Input: part model. Units: mm. Frame: model coordinates. Face numbers are marked on the shaded views. A direction names the side the tool comes from. Give positions to 0.01 mm unless a question says otherwise; leave off trailing zeros. Loops run counter-clockwise (first coordinate to the right, second up) from the corner with the lowest first, then second, coordinate; pieces in that order, holes last. Notation, with made-up numbers: (61, -23.75) -> (96, -23.75) arc R24 cw to (96, -11.75) -> close; hole circle Ø2 at (81, 3). An arc over 180 degrees is marked (long way). One line per question, with ' | ' between items.
from build123d import *

# Parameters (mm, degrees)
CIRPATTERN1_COUNT = 6


with BuildPart() as part:
    # Sketch1 → Revolve1 (revolve)
    with BuildSketch(Plane.XY, mode=Mode.PRIVATE) as revolve1_sk:
        Polygon((0, 16), (0, 20), (7.5, 20), (7.5, 18.5), (13, 18.5), (13, 16), (13.5, 16), (13.5, 15), (29.4, 15), (29.4, 13.95), (30.8, 13.95), (30.8, 14.8), (32.2, 14.8), (32.2, 12), (7, 12), (7, 15), (6.5, 15), (6.5, 16), align=None)
    revolve(revolve1_sk.sketch.rotate(Axis((-3.70841034, 0, 0), (1, 0, 0)), 180), axis=Axis((-3.70841034, 0, 0), (1, 0, 0)))

    # Sketch4 → M3 Tapped Hole1 (revolve, cut)
    with BuildSketch(Plane(origin=(0, 0, 18), x_dir=(0, 0, 1), z_dir=(0, 1, 0))):
        Polygon((0, 0), (0, 8.251075774), (1.25, 7.5), (1.25, 0), align=None)
    m3_tapped_hole1 = revolve(axis=Axis((-6.35, 0, 18), (1, 0, 0)), mode=Mode.SUBTRACT)

    # CirPattern1: M3 Tapped Hole1 ×6 about axis
    cirpattern1_axis = Axis((0, 0, 0), (1, 0, 0))
    for i in range(1, CIRPATTERN1_COUNT):
        add(m3_tapped_hole1.rotate(cirpattern1_axis, i * 360 / CIRPATTERN1_COUNT), mode=Mode.SUBTRACT)


solid = part.part
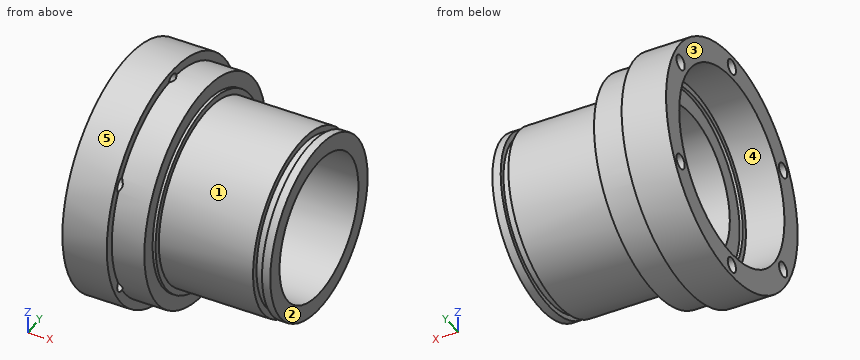
1. Section query A-A (x = 27.5). Output: boundary loops of the cut face in (y, z).
Determined:
outline: circle Ø30 at (0, 0); hole circle Ø24 at (0, 0)
2. Pull-direction query (Y, two-part tool) for the marked faces 3, 4 and 5; classes: pulls with the +Y half, pulls with the -Y half, needs draft (parallel to the pull), parting line crosses it, or undercut.
Determined:
face 3: needs draft | face 4: undercut | face 5: parting line crosses it
3. Pin query (flat end, axial travel): P1, Ø5, axis at x = 8.5, z = 9, coming from the +Y side; P2, Ø1.5, axis at y = -15.59, z = -9, coming from the +X side; P3, Ø4, axis at y = -11.5, z = -3, coming from the -X side. Return the tip coordinate at first contact, or that it passes through.
Determined:
P1: stops at y = 18.84 | P2: stops at x = 13 | P3: stops at x = 7
4. Reachability of the marked faces 1 and 2 from +Z, -Z, +X, -X, +Y, -Y: full face, straight path, thin tool, end or side. Return the list, or none.
Determined:
face 1: +X | face 2: +Z, -Z, +X, +Y, -Y
5. Section query C-C (x = 9.5). Output: boundary loops of the cut face in (y, z), then the cut area to 3 significant figures.
Determined:
outline: circle Ø37 at (0, 0); hole circle Ø24 at (0, 0) | area: 623 mm2
6. Ray query, line 1 along Z through (x, y) = (6, 0); line 2 along Y through (x, z) = (1.75, 9); line 3 along X through (y, z) = (-12.5, -5). Return the intervals inside material, ascending. Write a range as from..to.
Determined:
line 1: z = -20..-19.25, -16.75..-16, 16..16.75, 19.25..20 | line 2: y = -17.86..-16.84, -14.34..-13.23, 13.23..14.34, 16.84..17.86 | line 3: x = 7..32.2
